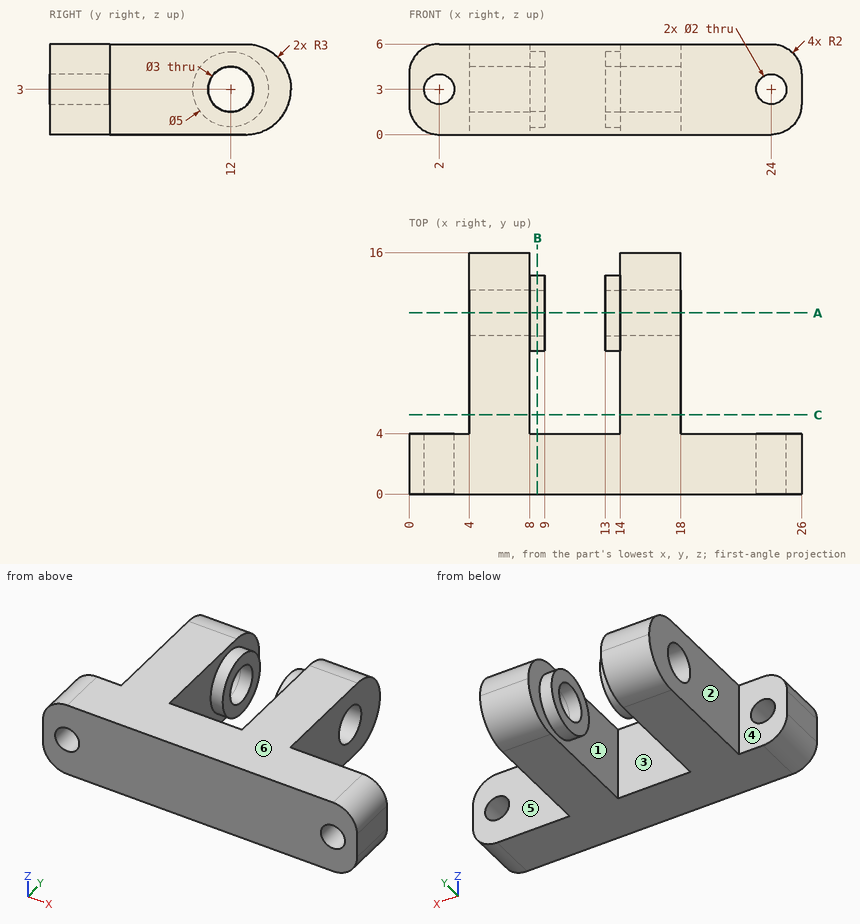
Verification items for this drawing (mm, ordinates from the low corner). A direction names the side the tool comes from. Round coordinates to 2 decimals unless told otherwise and drop trailing zeros. Write each loop counter-clockwise with the first axis right and the second up, starting at its lowest first coordinate (ties: lowest second). Pieces come first, ordered by that corner, then holes. Notation, with made-up numbers: M 25.5,71.5 L 34.5,71.5 A13 cw 34.5,85.5 Z; hole C 71,-1 d9. An arc over 180 degrees is marked long. Write item = value, one per line. Start each with the question number.
1. Scan lines: line 1 (X direction, y = 1.7, z = 3); line 2 (Y direction, x = 8.25, z = 3); line 3 (X direction, y = 6.5, z = 1.5). Record each from-to range of solid material in increasing order. Write a range as [from, to].
2. Tool access check on the marked faces 5 and 6. Record the directions out of +Z, -Z, +X, -X, +Y, -Y that give a thin tool (end or side, any length) a straight path to the whole face; none if there is none.
3. Release check for a two-part mould opening along X. For the marked faces 1, 2, 3 and 4 record: pulls with the +X half, pulls with the -X half, needs draft (parallel to the pull), parting line crosses it, or undercut.
4. Gauge pin test, flat ends, axial feed: pin 1 (3 mm diameter, centred on y = 9, z = 1.5, fed in from +X); pin 2 (3 mm diameter, centred on y = 9, z = 3.5, fed in from -X); pin 3 (1.8 mm diameter, centred on x = 21.5, z = 4.5, fed in from +Y). Record the tip position at first contact, or that the pin passes through.
5. Section check A-A, the plane y = 12. Record the cut outline in (x, z), then the cut area to 3 significant figures.
6. Section check B-B, the plane x = 8.5. Record the cut outline in (y, z), then the cut area to 3 significant figures.
7. Section check C-C, the plane y = 5.25. Record the cut outline in (x, z).
Results found:
q1.line_1 = [0, 1], [3, 23], [25, 26]
q1.line_2 = [0, 4], [9.5, 10.5], [13.5, 14.5]
q1.line_3 = [4, 8], [14, 18]
q2.face_5 = +Z, -Z, +X, +Y
q2.face_6 = +Z, +X, -X, +Y, -Y
q3.face_1 = undercut
q3.face_2 = pulls with the -X half
q3.face_3 = undercut
q3.face_4 = needs draft
q4.pin_1 = 18
q4.pin_2 = 4
q4.pin_3 = 4
q5.outline = M 4,0 L 8,0 L 8,0.5 L 9,0.5 L 9,1.5 L 4,1.5 Z; M 4,4.5 L 9,4.5 L 9,5.5 L 8,5.5 L 8,6 L 4,6 Z; M 13,0.5 L 14,0.5 L 14,0 L 18,0 L 18,1.5 L 13,1.5 Z; M 13,4.5 L 18,4.5 L 18,6 L 14,6 L 14,5.5 L 13,5.5 Z
q5.area = 28.0 mm^2
q6.outline = M 0,0 L 4,0 L 4,6 L 0,6 Z; C 12,3 d5; hole C 12,3 d3
q6.area = 36.6 mm^2
q7.outline = M 4,0 L 8,0 L 8,6 L 4,6 Z; M 14,0 L 18,0 L 18,6 L 14,6 Z
